```python
from build123d import *

# Parameters (mm, degrees)
F0_W         = 18
F0_H         = 60
F0_R         = 1.5
F1_DEPTH     = 15
F3_DEPTH     = 80
F4_W         = 12.820621879
F4_H         = 54.2796626687
F5_DEPTH     = 25
F6_R         = 1
F7_T4_DEPTH  = 18
F7_T10_DEPTH = 18
F7_T16_DEPTH = 18
F7_T22_DEPTH = 18
F7_T28_DEPTH = 18
F7_T34_DEPTH = 18
F7_T37_DEPTH = 43


# Not quite as in the source:
# - a fillet or chamfer that OpenCascade refuses, or shapes differently, is made with other operations: its cross-section is extruded or revolved along the edge and cut away or added


with BuildPart() as f1:
    # F0 (on Right) → F1 (new body)
    with BuildSketch(Plane.YZ):
        Rectangle(F0_W, F0_H)
        with Locations((0, -15)):
            Circle(F0_R, mode=Mode.SUBTRACT)
        with Locations((0, 15)):
            Circle(F0_R, mode=Mode.SUBTRACT)
    extrude(amount=F1_DEPTH)

    # F2 (on face) → F3 (cut)
    with BuildSketch(Plane.XY.offset(30)):
        Polygon((15, -9), (15, 9), (6, 0), align=None)
    extrude(amount=-F3_DEPTH, mode=Mode.SUBTRACT)

    # F4 (on face) → F5 (cut)
    with BuildSketch(Plane.XZ.offset(9)):
        with Locations((8.5896890605, 0)):
            Rectangle(F4_W, F4_H)
    extrude(amount=-F5_DEPTH, mode=Mode.SUBTRACT)

    # F6
    f6_edges = [f1.edges().sort_by_distance(p)[0] for p in [
        (15, -9, 28.569916),
        (15, 9, 28.569916),
        (15, -9, -28.569916),
        (15, 9, -28.569916),
    ]]
    fillet(f6_edges, radius=F6_R)

    # F7: fillet of radius 5 on 4 edges, made by hand


with BuildPart() as f7_tool2:
    # F7_s3 → F7_t4 (new body)
    with BuildSketch(Plane.XZ.offset(9)):
        with BuildLine():
            ThreePointArc((7.179378121, 27.1398313344), (3.6438442151, 25.6753652403), (2.179378121, 22.1398313344))
            Line((2.179378121, 22.1398313344), (2.179378121, 27.1398313344))
            Line((2.179378121, 27.1398313344), (7.179378121, 27.1398313344))
        make_face()
    extrude(amount=-F7_T4_DEPTH)

    split(bisect_by=Plane(origin=(3, 3, 0), x_dir=(0, 0, 1), z_dir=(-0.7071067812, -0.7071067812, 0)), keep=Keep.TOP)

    split(bisect_by=Plane(origin=(3, -3, 0), x_dir=(0, 0, 1), z_dir=(0.7071067812, -0.7071067812, 0)), keep=Keep.TOP)


with BuildPart() as f1_1:
    add(f1.part)

    # F7_t1: union F7_tool2
    add(f7_tool2.part)


with BuildPart() as f7_tool8:
    # F7_s9 → F7_t10 (new body)
    with BuildSketch(Plane.XZ.offset(9)):
        with BuildLine():
            ThreePointArc((7.179378121, 27.1398313344), (3.6438442151, 25.6753652403), (2.179378121, 22.1398313344))
            Line((2.179378121, 22.1398313344), (2.179378121, 27.1398313344))
            Line((2.179378121, 27.1398313344), (7.179378121, 27.1398313344))
        make_face()
    extrude(amount=-F7_T10_DEPTH)

    split(bisect_by=Plane(origin=(3, 3, 0), x_dir=(0, 0, 1), z_dir=(-0.7071067812, -0.7071067812, 0)), keep=Keep.TOP)

    split(bisect_by=Plane(origin=(3, -3, 0), x_dir=(0, 0, 1), z_dir=(-0.7071067812, 0.7071067812, 0)), keep=Keep.TOP)


with BuildPart() as f1_2:
    add(f1_1.part)

    # F7_t7: union F7_tool8
    add(f7_tool8.part)


with BuildPart() as f7_tool14:
    # F7_s15 → F7_t16 (new body)
    with BuildSketch(Plane.XZ.offset(9)):
        with BuildLine():
            ThreePointArc((7.179378121, 27.1398313344), (3.6438442151, 25.6753652403), (2.179378121, 22.1398313344))
            Line((2.179378121, 22.1398313344), (2.179378121, 27.1398313344))
            Line((2.179378121, 27.1398313344), (7.179378121, 27.1398313344))
        make_face()
    extrude(amount=-F7_T16_DEPTH)

    split(bisect_by=Plane(origin=(3, 3, 0), x_dir=(0, 0, 1), z_dir=(0.7071067812, 0.7071067812, 0)), keep=Keep.TOP)

    split(bisect_by=Plane(origin=(3, -3, 0), x_dir=(0, 0, 1), z_dir=(-0.7071067812, 0.7071067812, 0)), keep=Keep.TOP)


with BuildPart() as f1_3:
    add(f1_2.part)

    # F7_t13: union F7_tool14
    add(f7_tool14.part)


with BuildPart() as f7_tool20:
    # F7_s21 → F7_t22 (new body)
    with BuildSketch(Plane.XZ.offset(9)):
        with BuildLine():
            ThreePointArc((2.179378121, -22.1398313344), (3.6438442151, -25.6753652403), (7.179378121, -27.1398313344))
            Line((7.179378121, -27.1398313344), (2.179378121, -27.1398313344))
            Line((2.179378121, -27.1398313344), (2.179378121, -22.1398313344))
        make_face()
    extrude(amount=-F7_T22_DEPTH)

    split(bisect_by=Plane(origin=(3, 3, 0), x_dir=(0, 0, 1), z_dir=(-0.7071067812, -0.7071067812, 0)), keep=Keep.TOP)

    split(bisect_by=Plane(origin=(3, -3, 0), x_dir=(0, 0, 1), z_dir=(0.7071067812, -0.7071067812, 0)), keep=Keep.TOP)


with BuildPart() as f1_4:
    add(f1_3.part)

    # F7_t19: union F7_tool20
    add(f7_tool20.part)


with BuildPart() as f7_tool26:
    # F7_s27 → F7_t28 (new body)
    with BuildSketch(Plane.XZ.offset(9)):
        with BuildLine():
            ThreePointArc((2.179378121, -22.1398313344), (3.6438442151, -25.6753652403), (7.179378121, -27.1398313344))
            Line((7.179378121, -27.1398313344), (2.179378121, -27.1398313344))
            Line((2.179378121, -27.1398313344), (2.179378121, -22.1398313344))
        make_face()
    extrude(amount=-F7_T28_DEPTH)

    split(bisect_by=Plane(origin=(3, 3, 0), x_dir=(0, 0, 1), z_dir=(-0.7071067812, -0.7071067812, 0)), keep=Keep.TOP)

    split(bisect_by=Plane(origin=(3, -3, 0), x_dir=(0, 0, 1), z_dir=(-0.7071067812, 0.7071067812, 0)), keep=Keep.TOP)


with BuildPart() as f1_5:
    add(f1_4.part)

    # F7_t25: union F7_tool26
    add(f7_tool26.part)


with BuildPart() as f7_tool32:
    # F7_s33 → F7_t34 (new body)
    with BuildSketch(Plane.XZ.offset(9)):
        with BuildLine():
            ThreePointArc((2.179378121, -22.1398313344), (3.6438442151, -25.6753652403), (7.179378121, -27.1398313344))
            Line((7.179378121, -27.1398313344), (2.179378121, -27.1398313344))
            Line((2.179378121, -27.1398313344), (2.179378121, -22.1398313344))
        make_face()
    extrude(amount=-F7_T34_DEPTH)

    split(bisect_by=Plane(origin=(3, 3, 0), x_dir=(0, 0, 1), z_dir=(0.7071067812, 0.7071067812, 0)), keep=Keep.TOP)

    split(bisect_by=Plane(origin=(3, -3, 0), x_dir=(0, 0, 1), z_dir=(-0.7071067812, 0.7071067812, 0)), keep=Keep.TOP)


with BuildPart() as f1_6:
    add(f1_5.part)

    # F7_t31: union F7_tool32
    add(f7_tool32.part)

    # F7_s38 → F7_t37 (cut)
    with BuildSketch(Plane.XZ.offset(-21.5)):
        with BuildLine():
            ThreePointArc((0, 25), (1.4644660941, 28.5355339059), (5, 30))
            Line((5, 30), (0, 30))
            Line((0, 30), (0, 25))
        make_face()
        with BuildLine():
            ThreePointArc((5, -30), (1.4644660941, -28.5355339059), (0, -25))
            Line((0, -25), (0, -30))
            Line((0, -30), (5, -30))
        make_face()
    extrude(amount=F7_T37_DEPTH, mode=Mode.SUBTRACT)


solid = f1_6.part
```
Work out the finished part from the listing and answer in its coordinate system (mm). A direction names the side the tool comes from. Coordinates: 2 decimals unless noted, no trailing zeros. Loops run counter-clockwise (first coordinate to the right, second up) from the corner with the lowest first, then second, coordinate; pieces in that order, holes last. Notation, with made-up numbers: (83.25, 53) -> (94.25, 53) arc R16 ccw to (94.25, 77) -> close; hole circle Ø8 at (-24, -35). An arc over 180 degrees is marked (long way). Answer as CSV lines item,"result".
Q1. A tool of negligible diameter and unlimited length cuts with its end or side. For faces 1 (the face through (7, -2, -30)), 2 (the face through (10, -4, 28)), 3 (the face through (4, 0, 26)), from which of +Z, -Z, +X, -X, +Y, -Y can it reach the whole face along a straight path? Write none if from no direction.
Findings:
face 1,"-Z, +X, -X, +Y, -Y"
face 2,"+Z, -Z, +X"
face 3,"+X, +Y, -Y"
Q2. The part is cut by section B-B on x = 10.5. Write down the section's boundary in (y, z).
Findings:
outline,"(-9, -30) -> (-4.5, -30) -> (-4.5, -27.14) -> (-9, -27.14) -> close; (-9, 27.14) -> (-4.5, 27.14) -> (-4.5, 30) -> (-9, 30) -> close; (4.5, -30) -> (9, -30) -> (9, -27.14) -> (4.5, -27.14) -> close; (4.5, 27.14) -> (9, 27.14) -> (9, 30) -> (4.5, 30) -> close"
Q3. For a pull along Y with two mould halves and no side action, classify faces 4 (the face through (7, -2, 30)), 5 (the face through (1.07, -1.11, 16.01)), 6 (the face through (2, -9, -7)), 7 (the face through (13.503, -8.398, 28.59)) as +Y half, -Y half, draft (parallel to the pull), parting line (faces both ways), or undercut.
Findings:
face 4,"draft"
face 5,"undercut"
face 6,"-Y half"
face 7,"undercut"
Q4. The part is cut by section D-D on y = -5.75. Write down the section's boundary in (x, z).
Findings:
outline,"(0, -25) arc R5 ccw to (5, -30) -> (11.75, -30) -> (11.75, -27.14) -> (7.18, -27.14) arc R5 cw to (2.18, -22.14) -> (2.18, 22.14) arc R5 cw to (7.18, 27.14) -> (11.75, 27.14) -> (11.75, 30) -> (5, 30) arc R5 ccw to (0, 25) -> close"
Q5. The part is cut by section C-C on y = 2.5. Write down the section's boundary in (x, z), and give its area (3 significant figures).
Findings:
outline,"(0, -25) arc R5 ccw to (5, -30) -> (8.5, -30) -> (8.5, -27.14) -> (7.18, -27.14) arc R5 cw to (2.18, -22.14) -> (2.18, 22.14) arc R5 cw to (7.18, 27.14) -> (8.5, 27.14) -> (8.5, 30) -> (5, 30) arc R5 ccw to (0, 25) -> close"
area,"167 mm²"
Q6. The part is cut by section A-A on z = -15. Write down the section's boundary in (x, y).
Findings:
outline,"(0, -9) -> (2.18, -9) -> (2.18, -1.5) -> (0, -1.5) -> close; (0, 1.5) -> (2.18, 1.5) -> (2.18, 9) -> (0, 9) -> close"
Q7. Find the intervals of material crossed by probe 1 along Y at (x, z) = (1.2, -15); probe 2 along X at (y, z) = (-2.25, 2.5); probe 3 along Z at (x, y) = (11, 7.5), in increasing order.
Findings:
probe 1,"y = -9 to -1.5, 1.5 to 9"
probe 2,"x = 0 to 2.18"
probe 3,"z = -30 to -27.14, 27.14 to 30"
Q8. Each of these flat-tipped pins is pushed along its axis until it touches: pin 1 (1 mm diameter, centred on x = 3, z = -16.5, fed in from +Y); pin 2 (5 mm diameter, centred on y = 0, z = -15, fed in from -X); pin 3 (1.5 mm diameter, centred on x = 2, y = -1.5, fed in from -Z); pin 4 (9 mm diameter, centred on y = -4.5, z = 4.5, fed in from +X). Where does it stop, or does it pass through?
Findings:
pin 1,"passes through"
pin 2,"stops at x = 0"
pin 3,"stops at z = -29.47"
pin 4,"stops at x = 2.18"
